```python
from build123d import *

# Parameters (mm, degrees)
F1_DEPTH = 20
F2_R     = 6
F3_R     = 1.917143
F4_DEPTH = 25
F6_DEPTH = 20
F8_DEPTH = 12.5


with BuildPart() as f1:
    # F0 (on Front) → F1 (new body)
    with BuildSketch(Plane.XZ):
        with BuildLine():
            Line((-25, 3), (-25, 0))
            Line((-25, 0), (-13.5, 0))
            ThreePointArc((-13.5, 0), (0, 13.5), (13.5, 0))
            Line((13.5, 0), (25, 0))
            Line((25, 0), (25, 3))
            Line((25, 3), (16.224981, 3))
            ThreePointArc((16.224981, 3), (0, 16.5), (-16.224981, 3))
            Line((-16.224981, 3), (-25, 3))
        make_face()
    extrude(amount=F1_DEPTH)

    # F2
    f2_edges = [f1.edges().sort_by_distance(p)[0] for p in [
        (25, -20, 1.5),
        (25, 0, 1.5),
        (-25, -20, 1.5),
        (-25, 0, 1.5),
    ]]
    fillet(f2_edges, radius=F2_R)

    # F3 (on face) → F4 (cut)
    with BuildSketch(Plane.XY.offset(3)):
        with Locations((-21, -10)):
            Circle(F3_R)
        with Locations((21, -10)):
            Circle(F3_R)
    extrude(amount=-F4_DEPTH, mode=Mode.SUBTRACT)

    # F5 (on Front) → F6 (join)
    with BuildSketch(Plane.XZ):
        with BuildLine():
            Line((12, 20), (-12, 20))
            Line((-12, 20), (-12, 10.583005))
            ThreePointArc((-12, 10.583005), (0, 16), (12, 10.583005))
            Line((12, 10.583005), (12, 20))
        make_face()
    extrude(amount=F6_DEPTH)

    # F7 (on Right) → F8 (cut, symmetric)
    with BuildSketch(Plane.YZ):
        Polygon((-12, 20), (-15, 20), (-15, 18.2), (-18, 18.2), (-18, 16.4), (-12, 16.4), align=None)
        Polygon((-5, 20), (-8, 20), (-8, 16.4), (-2, 16.4), (-2, 18.2), (-5, 18.2), align=None)
    extrude(amount=F8_DEPTH, both=True, mode=Mode.SUBTRACT)


solid = f1.part
```
Could you check a few things on this model? Use its own coordinates, in mm. A direction names the side the tool comes from. Round coordinates to 2 decimals unless told otherwise and drop trailing zeros. Loops run counter-clockwise (first coordinate to the right, second up) from the corner with the lowest first, then second, coordinate; pieces in that order, holes last. Notation, with made-up numbers: M -35.5,0.5 L -25.5,0.5 A5 cw -25.5,7.5 Z; hole C -10.5,-37.5 d9. An arc over 180 degrees is marked long. Answer as CSV lines item,"result".
1) Imagine slicing it at B-B on y = -16. List the corners of the cut face in (x, z) for me, and give its area (3 significant figures).
From the geometry:
outline,"M -24.66,0 L -13.5,0 A13.5 cw 13.5,0 L 24.66,0 L 24.66,3 L 16.22,3 A16.5 ccw 12,11.32 L 12,16.4 L -12,16.4 L -12,11.32 A16.5 ccw -16.22,3 L -24.66,3 Z; M -12,18.2 L 12,18.2 L 12,20 L -12,20 Z"
area,"270 mm^2"
2) We'd pull the mould along Z, two halves only. Please class faces 4 (the flat face through (18.7, -9.9, 3)), 5 (the flat face through (0, -15, 16.4)), 6 (the flat face through (0, -3, 18.2)), 7 (the flat face through (0, -12, 18)): released by +Z, released by -Z, zero draft, split by the parting line, or undercut.
From the geometry:
face 4,"released by +Z"
face 5,"undercut"
face 6,"undercut"
face 7,"zero draft"
3) For pin 1 Ø4.5 at (x, y) = (-22, -6) entering from +Z; pin 2 Ø3.5 at (x, y) = (-1, -3) entering from -Z; pin 3 Ø3 at (x, y) = (-21, -10) entering from -Z; pin 4 Ø3 at (y, z) = (-3, 18) entering from +X, each with a flat end and sliding along its axis, tell me the tip position at first contact or that it passes through.
From the geometry:
pin 1,"z = 3"
pin 2,"z = 13.22"
pin 3,"through"
pin 4,"x = 12"
4) Which directions (+Z, -Z, +X, -X, +Y, -Y) give clear straight access to the entire face, cutting with the end or side of a thin tool? Please do faces 1 (the flat face through (0, -5, 19)), 2 (the flat face through (0, -18, 17)), 3 (the flat face through (-12, -10, 15)).
From the geometry:
face 1,"+Z, +X, -X"
face 2,"+X, -X"
face 3,"+Z, -X, +Y, -Y"
5) If I drill on probe 1 along X at (y, z) = (-8.75, 19); probe 2 along Y at (x, z) = (-21, 2.2); probe 3 along Z at (x, y) = (18, -16), over which ranges is the centre line in solid material (lowest first)?
From the geometry:
probe 1,"-12 to 12"
probe 2,"-19.66 to -11.92, -8.08 to -0.34"
probe 3,"0 to 3"
6) Imagine slicing it at A-A on x = 21. List the corners of the cut face in (y, z) for me.
From the geometry:
outline,"M -19.66,0 L -11.92,0 L -11.92,3 L -19.66,3 Z; M -8.08,0 L -0.34,0 L -0.34,3 L -8.08,3 Z"
7) Imagine slicing it at D-D on x = 0. List the corners of the cut face in (y, z) for me, and give its area (3 significant figures).
From the geometry:
outline,"M -20,13.5 L 0,13.5 L 0,20 L -5,20 L -5,18.2 L -2,18.2 L -2,16.4 L -8,16.4 L -8,20 L -12,20 L -12,16.4 L -18,16.4 L -18,18.2 L -15,18.2 L -15,20 L -20,20 Z"
area,"97.6 mm^2"
8) Imagine slicing it at C-C on z = 10.5. List the corners of the cut face in (x, y) for me.
From the geometry:
outline,"M -12.73,-20 L -8.49,-20 L -8.49,0 L -12.73,0 Z; M 8.49,-20 L 12.73,-20 L 12.73,0 L 8.49,0 Z"
